Verification items for this drawing (mm, ordinates from the low corner). Coordinates: 2 decimals unless noted, no trailing zeros. Write each loop counter-clockwise with the first axis right and the second up, starting at its lowest first coordinate (ties: lowest second). Pieces come first, ordered by that corner, then holes.
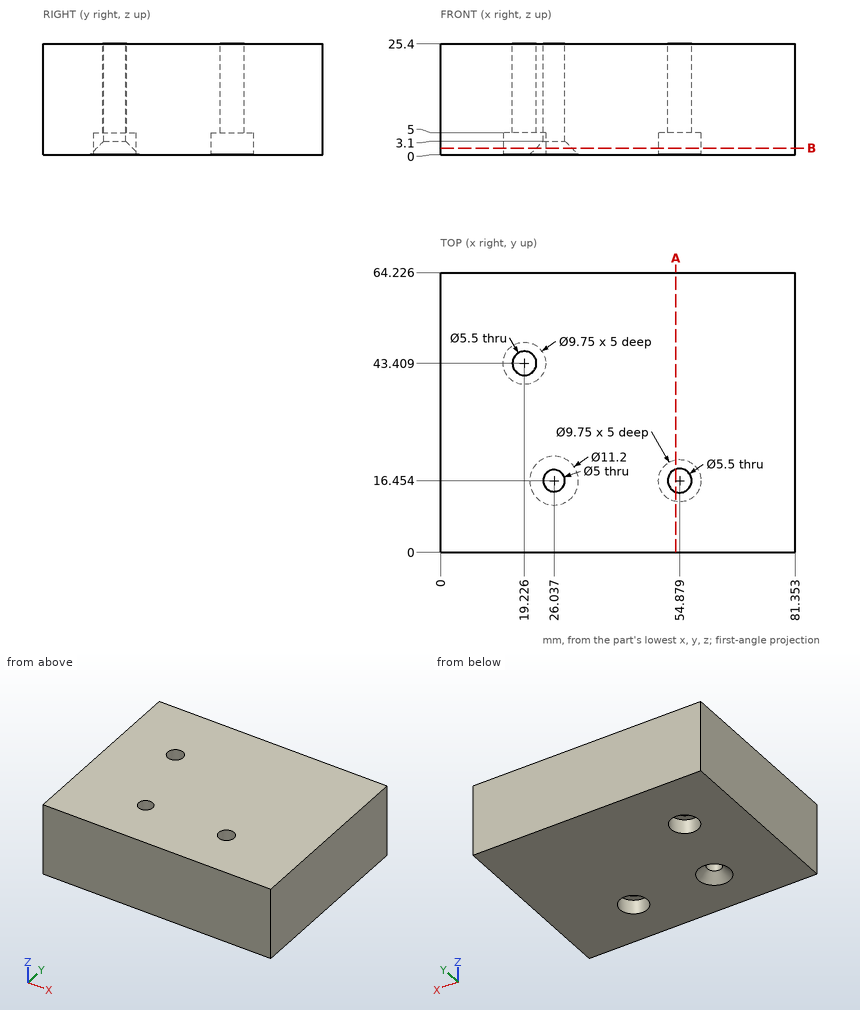
1. Sectioned sample at B-B, the plane z = 1.5. Give the number of separate pieces and of enclosed holes in the cut face, and give its area (3 significant figures).
Computed values:
separate pieces: 1
enclosed holes: 3
area: 5,020 mm2
2. Gauge pin test, flat end, axial feed: pin 1 Ø3.5 at (x, y) = (19.23, 43.41) entering from +Z. Record the tip position at first contact, or that the pin passes through.
Computed values:
pin 1: passes through
3. Thickness scan on line 1 along Y through (x, z) = (20.5, 5.5) (1 decimal); line 2 along X through (y, z) = (42, 15.75) (1 decimal); line 3 along Z through (x, y) = (27, 12) (1 decimal). Record the ranges inside material, lowest first.
Computed values:
line 1: y = 0 to 41, 45.8 to 64.2
line 2: x = 0 to 16.9, 21.6 to 81.4
line 3: z = 1 to 25.4
4. Sectioned sample at A-A, the plane x = 54. Record the boundary of the cut face in (y, z).
Computed values:
outline: (0, 0) - (11.66, 0) - (11.66, 5) - (13.85, 5) - (13.85, 25.4) - (0, 25.4) - close; (19.06, 5) - (21.25, 5) - (21.25, 0) - (64.23, 0) - (64.23, 25.4) - (19.06, 25.4) - close
